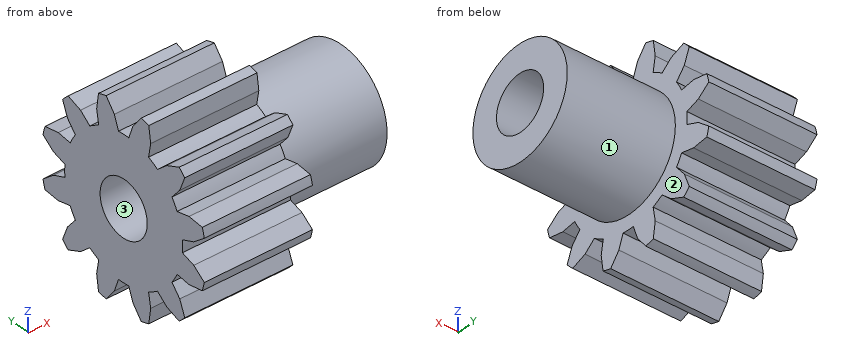
Autodesk Inventor part; units mm, degrees
ref_plane "YZ Plane" through (0, 0, 0) normal (1, 0, 0) x (0, 1, 0)
ref_plane "XZ Plane" through (0, 0, 0) normal (0, 1, 0) x (-1, 0, 0)
ref_plane "XY Plane" through (0, 0, 0) normal (0, 0, 1) x (1, 0, 0)
sketch "Skizze_1" plane through (0, 0, 0) normal (1, 0, 0) x (0, 1, 0)
  arc A0 (-0.7439, 3.42) -> (-1.0658, 3.3338) centre (0, 0) ccw
  line L0 (-1.0658, 3.3338) -> (-1.1459, 2.7725)
  line L1 (-1.1459, 2.7725) -> (-1.0565, 2.2658)
  arc A1 (-1.0565, 2.2658) -> (-1.4339, 2.0479) centre (0, 0) ccw
  line L2 (-1.4339, 2.0479) -> (-1.8281, 2.3786)
  line L3 (-1.8281, 2.3786) -> (-2.3542, 2.5899)
  arc A2 (-2.3542, 2.5899) -> (-2.5899, 2.3542) centre (0, 0) ccw
  line L4 (-2.5899, 2.3542) -> (-2.3786, 1.8281)
  line L5 (-2.3786, 1.8281) -> (-2.0479, 1.4339)
  arc A3 (-2.0479, 1.4339) -> (-2.2658, 1.0565) centre (0, 0) ccw
  line L6 (-2.2658, 1.0565) -> (-2.7725, 1.1459)
  line L7 (-2.7725, 1.1459) -> (-3.3338, 1.0658)
  arc A4 (-3.3338, 1.0658) -> (-3.42, 0.7439) centre (0, 0) ccw
  line L8 (-3.42, 0.7439) -> (-2.974, 0.3939)
  line L9 (-2.974, 0.3939) -> (-2.4905, 0.2179)
  arc A5 (-2.4905, 0.2179) -> (-2.4905, -0.2179) centre (0, 0) ccw
  line L10 (-2.4905, -0.2179) -> (-2.974, -0.3939)
  line L11 (-2.974, -0.3939) -> (-3.42, -0.7439)
  arc A6 (-3.42, -0.7439) -> (-3.3338, -1.0658) centre (0, 0) ccw
  line L12 (-3.3338, -1.0658) -> (-2.7725, -1.1459)
  line L13 (-2.7725, -1.1459) -> (-2.2658, -1.0565)
  arc A7 (-2.2658, -1.0565) -> (-2.0479, -1.4339) centre (0, 0) ccw
  line L14 (-2.0479, -1.4339) -> (-2.3786, -1.8281)
  line L15 (-2.3786, -1.8281) -> (-2.5899, -2.3542)
  arc A8 (-2.5899, -2.3542) -> (-2.3542, -2.5899) centre (0, 0) ccw
  line L16 (-2.3542, -2.5899) -> (-1.8281, -2.3786)
  line L17 (-1.8281, -2.3786) -> (-1.4339, -2.0479)
  arc A9 (-1.4339, -2.0479) -> (-1.0565, -2.2658) centre (0, 0) ccw
  line L18 (-1.0565, -2.2658) -> (-1.1459, -2.7725)
  line L19 (-1.1459, -2.7725) -> (-1.0658, -3.3338)
  arc A10 (-1.0658, -3.3338) -> (-0.7439, -3.42) centre (0, 0) ccw
  line L20 (-0.7439, -3.42) -> (-0.3939, -2.974)
  line L21 (-0.3939, -2.974) -> (-0.2179, -2.4905)
  arc A11 (-0.2179, -2.4905) -> (0.2179, -2.4905) centre (0, 0) ccw
  line L22 (0.2179, -2.4905) -> (0.3939, -2.974)
  line L23 (0.3939, -2.974) -> (0.7439, -3.42)
  arc A12 (0.7439, -3.42) -> (1.0658, -3.3338) centre (0, 0) ccw
  line L24 (1.0658, -3.3338) -> (1.1459, -2.7725)
  line L25 (1.1459, -2.7725) -> (1.0565, -2.2658)
  arc A13 (1.0565, -2.2658) -> (1.4339, -2.0479) centre (0, 0) ccw
  line L26 (1.4339, -2.0479) -> (1.8281, -2.3786)
  line L27 (1.8281, -2.3786) -> (2.3542, -2.5899)
  arc A14 (2.3542, -2.5899) -> (2.5899, -2.3542) centre (0, 0) ccw
  line L28 (2.5899, -2.3542) -> (2.3786, -1.8281)
  line L29 (2.3786, -1.8281) -> (2.0479, -1.4339)
  arc A15 (2.0479, -1.4339) -> (2.2658, -1.0565) centre (0, 0) ccw
  line L30 (2.2658, -1.0565) -> (2.7725, -1.1459)
  line L31 (2.7725, -1.1459) -> (3.3338, -1.0658)
  arc A16 (3.3338, -1.0658) -> (3.42, -0.7439) centre (0, 0) ccw
  line L32 (3.42, -0.7439) -> (2.974, -0.3939)
  line L33 (2.974, -0.3939) -> (2.4905, -0.2179)
  arc A17 (2.4905, -0.2179) -> (2.4905, 0.2179) centre (0, 0) ccw
  line L34 (2.4905, 0.2179) -> (2.974, 0.3939)
  line L35 (2.974, 0.3939) -> (3.42, 0.7439)
  arc A18 (3.42, 0.7439) -> (3.3338, 1.0658) centre (0, 0) ccw
  line L36 (3.3338, 1.0658) -> (2.7725, 1.1459)
  line L37 (2.7725, 1.1459) -> (2.2658, 1.0565)
  arc A19 (2.2658, 1.0565) -> (2.0479, 1.4339) centre (0, 0) ccw
  line L38 (2.0479, 1.4339) -> (2.3786, 1.8281)
  line L39 (2.3786, 1.8281) -> (2.5899, 2.3542)
  arc A20 (2.5899, 2.3542) -> (2.3542, 2.5899) centre (0, 0) ccw
  line L40 (2.3542, 2.5899) -> (1.8281, 2.3786)
  line L41 (1.8281, 2.3786) -> (1.4339, 2.0479)
  arc A21 (1.4339, 2.0479) -> (1.0565, 2.2658) centre (0, 0) ccw
  line L42 (1.0565, 2.2658) -> (1.1459, 2.7725)
  line L43 (1.1459, 2.7725) -> (1.0658, 3.3338)
  arc A22 (1.0658, 3.3338) -> (0.7439, 3.42) centre (0, 0) ccw
  line L44 (0.7439, 3.42) -> (0.3939, 2.974)
  line L45 (0.3939, 2.974) -> (0.2179, 2.4905)
  arc A23 (0.2179, 2.4905) -> (-0.2179, 2.4905) centre (0, 0) ccw
  line L46 (-0.2179, 2.4905) -> (-0.3939, 2.974)
  line L47 (-0.3939, 2.974) -> (-0.7439, 3.42)
extrude "Extrusion1" add sketch "Skizze_1" along normal mid plane 4
sketch "Skizze_2" plane through (0, 0, 0) normal (0, 0, 1) x (1, 0, 0)
  line L0 (6, 0) -> (2, 0)
  line L1 (2, 0) -> (2, 2)
  line L2 (2, 2) -> (6, 2)
  line L3 (6, 2) -> (6, 0)
  line L4 (6, 0) -> (2, 0)
revolve "Revolution1" add sketch "Skizze_2" angle 360 about axis through (6, 0, 0) along (1, 0, 0)
sketch "Skizze_3" plane through (6, 0, 0) normal (1, 0, 0) x (0, 1, 0)
  circle A0 centre (0, 0) radius 1
extrude "Extrusion2" cut sketch "Skizze_3" along normal mid plane 16
properties part number "M-0.5 Zb-4mm M-0.7 Zb-5mm mN 21101200"
Geometry: final body of the model. Coordinates: model frame, mm. Face numbers are marked on the shaded views. Give positions to 0.01 mm unless a question says otherwise; leave off trailing zeros. Write each loop counter-clockwise with the first axis right and the second up, starting at its lowest first coordinate (ties: lowest second). Pieces come first, ordered by that corner, then holes.
1. Line query: probe 1 along Z at (x, y) = (3.25, 0); probe 2 along Z at (x, y) = (0, 3); probe 3 along X at (y, z) = (1.75, 1.75). Output: solid intervals per line, ascending.
2. Section query D-D, the plane z = -1.25. Return loops of the section in (x, y).
3. Pin query (flat end, axial travel): P1, Ø1.5, axis at y = -2.5, z = -2, coming from the +X side; P2, Ø2, axis at x = 5, z = -1.5, coming from the -Y side. Return the tip coordinate at first contact, or that it passes through.
4. Draft query along Z for the marked faces 1, 2 and 3. Return one class per face: released by +Z, released by -Z, zero draft, split by the parting line, or undercut.
5. Section query C-C, the plane x = 3.5. Return loops of the section in (y, z), then the cut area to 3 significant figures.
6. Section query A-A, the plane z = 0. Return loops of the section in (x, y), then the cut area to 3 significant figures.
Computed:
1. probe 1: z = -2 to -1, 1 to 2
1. probe 2: z = -1.11 to -0.41, 0.41 to 1.11
1. probe 3: x = -2 to 2
2. outline: (-2, -2.17) - (2, -2.17) - (2, -1.56) - (6, -1.56) - (6, 1.56) - (2, 1.56) - (2, 2.17) - (-2, 2.17) - close
3. P1: stops at x = 2
3. P2: stops at y = -1.94
4. face 1: split by the parting line
4. face 2: zero draft
4. face 3: undercut
5. outline: circle Ø4 at (0, 0); hole circle Ø2 at (0, 0)
5. area: 9.42 mm2
6. outline: (-2, -2.5) - (2, -2.5) - (2, -2) - (6, -2) - (6, -1) - (-2, -1) - close; (-2, 1) - (6, 1) - (6, 2) - (2, 2) - (2, 2.5) - (-2, 2.5) - close
6. area: 20.0 mm2
